from build123d import *

# Parameters (mm, degrees)
F0_W            = 40
F0_H            = 20
F1_DEPTH        = 15
F2_R            = 2.5
F3_DEPTH        = 15.001
F4_W            = 7
F4_H            = 3.5
F5_DEPTH        = 14.5
F6_W            = 4
F6_H            = 2.5
F7_DEPTH        = 12.5
F7_COPIES_COUNT = 2
F7_COPIES_PITCH = 31.5
F8_T1_DEPTH     = 2.5
F9_T4_DEPTH     = 2.5
F9_S5_R         = 2.5
F9_T6_DEPTH     = 4


# Not quite as in the source:
# - a fillet or chamfer that OpenCascade refuses, or shapes differently, is made with other operations: its cross-section is extruded or revolved along the edge and cut away or added
# - a pattern or mirror of a feature is missing from the dataset's text; its kind, count and spacing are read off the source's solid


with BuildPart() as f1:
    # F0 (on Top) → F1 (new body)
    with BuildSketch(Plane.XY):
        Rectangle(F0_W, F0_H)
    extrude(amount=F1_DEPTH)

    # F2 (on face) → F3 (cut, through all)
    with BuildSketch(Plane.XY.offset(15)):
        with Locations((-10, 0)):
            Circle(F2_R)
        with Locations((10, 0)):
            Circle(F2_R)
    extrude(amount=-F3_DEPTH, mode=Mode.SUBTRACT)

    # F4 (on face) → F5 (cut)
    with BuildSketch(Plane(origin=(-20, 0, 0), x_dir=(0, -1, 0), z_dir=(-1, 0, 0))):
        with Locations((0, 4.25)):
            Rectangle(F4_W, F4_H)
        with Locations((0, 10.75)):
            Rectangle(F4_W, F4_H)
    f5 = extrude(amount=-F5_DEPTH, mode=Mode.SUBTRACT)

    # F5_copies: F5 across plane
    add(f5.mirror(Plane(origin=(0, 0, 0), x_dir=(0, 0, 1), z_dir=(1, 0, 0))), mode=Mode.SUBTRACT)

    # F6 (on face) → F7 (cut)
    with BuildSketch(Plane(origin=(-20, 0, 0), x_dir=(0, -1, 0), z_dir=(-1, 0, 0))):
        with Locations((0, 13.75)):
            Rectangle(F6_W, F6_H)
    f7 = extrude(amount=-F7_DEPTH, mode=Mode.SUBTRACT)

    # F7_copies: F7 ×2
    with Locations(*[(i * F7_COPIES_PITCH, 0, 0) for i in range(1, F7_COPIES_COUNT)]):
        add(f7, mode=Mode.SUBTRACT)

    # F8: fillet of radius 2.5 on 1 edges, made by hand

    # F8_s2 → F8_t1 (join)
    with BuildSketch(Plane.XY.offset(12.5)):
        with BuildLine():
            ThreePointArc((-8.5, -2), (-7.7639320225, -1.1180339887), (-7.5, 0))
            Line((-7.5, 0), (-7.5, -2))
            Line((-7.5, -2), (-8.5, -2))
        make_face()
    extrude(amount=F8_T1_DEPTH)

    # F9: fillet of radius 2.5 on 1 edges, made by hand


with BuildPart() as f9_tool2:
    # F9_s3 → F9_t4 (new body)
    with BuildSketch(Plane.XY.offset(15)):
        with BuildLine():
            ThreePointArc((-7.5, -0.5), (-8.232233047, 1.267766953), (-10, 2))
            Line((-10, 2), (-7.5, 2))
            Line((-7.5, 2), (-7.5, -0.5))
        make_face()
    extrude(amount=-F9_T4_DEPTH)

    # F9_s5 → F9_t6 (cut, symmetric)
    with BuildSketch(Plane.XY.offset(13.8)):
        with Locations((-10, 0)):
            Circle(F9_S5_R)
    extrude(amount=F9_T6_DEPTH, both=True, mode=Mode.SUBTRACT)


with BuildPart() as f1_1:
    add(f1.part)

    # F9_t1: union F9_tool2
    add(f9_tool2.part)


solid = f1_1.part
CAD build for the part. Positions are in the model's coordinates, mm. A direction names the side the tool comes from. Give positions to 0.01 mm unless a question says otherwise; leave off trailing zeros. Order: outer loops, then holes, each group sorted by start corner. A loop starts at its lowest first (then second) coordinate and runs counter-clockwise, first axis right, second up. Notation, with made-up numbers: (-22.75, -30) -> (-13.75, -30) arc R21 ccw to (-13.75, -24) -> close; hole circle Ø1 at (-0.75, 75). An arc over 180 degrees is marked (long way). Return JSON: item names as keys, results as strings.
Q1. Which spindle directions (+Z, -Z, +X, -X, +Y, -Y) get a long thin tool onto all of the face, cutting with end or side? Do faces 1 (the face through (13, 3.5, 11)), 2 (the face through (-13, 3.5, 11)), 3 (the face through (7.5, 0.1, 1.3)). Say none if no direction does.
Working result:
{"face 1": "+X", "face 2": "-X", "face 3": "+Z, -Z"}
Q2. Saw through at C-C (x = 17). Write the cut outline in (y, z).
Working result:
{"outline": "(-10, 0) -> (10, 0) -> (10, 15) -> (2, 15) -> (2, 12.5) -> (3.5, 12.5) -> (3.5, 9) -> (-3.5, 9) -> (-3.5, 12.5) -> (-2, 12.5) -> (-2, 15) -> (-10, 15) -> close; hole (-3.5, 2.5) -> (3.5, 2.5) -> (3.5, 6) -> (-3.5, 6) -> close"}
Q3. Saw through at D-D (z = 14.25). Write the cut outline in (x, y), then the cut area to 3 significant figures.
Working result:
{"outline": "(-20, -10) -> (20, -10) -> (20, -2) -> (11.5, -2) arc R2.5 cw (long way) to (11.5, 2) -> (20, 2) -> (20, 10) -> (-20, 10) -> (-20, 2) -> (-11.5, 2) arc R2.5 cw (long way) to (-11.5, -2) -> (-20, -2) -> close", "area": "698 mm²"}
Q4. Saw through at B-B (z = 2). Write the cut outline in (x, y), then the cut area to 3 significant figures.
Working result:
{"outline": "(-20, -10) -> (20, -10) -> (20, 10) -> (-20, 10) -> close; hole circle Ø5 at (-10, 0); hole circle Ø5 at (10, 0)", "area": "761 mm²"}
Q5. Saw through at A-A (x = -10). Write the cut outline in (y, z).
Working result:
{"outline": "(-10, 0) -> (-2.5, 0) -> (-2.5, 2.5) -> (-3.5, 2.5) -> (-3.5, 6) -> (-2.5, 6) -> (-2.5, 9) -> (-3.5, 9) -> (-3.5, 12.5) -> (-2.5, 12.5) -> (-2.5, 15) -> (-10, 15) -> close; (2.5, 0) -> (10, 0) -> (10, 15) -> (2.5, 15) -> (2.5, 12.5) -> (3.5, 12.5) -> (3.5, 9) -> (2.5, 9) -> (2.5, 6) -> (3.5, 6) -> (3.5, 2.5) -> (2.5, 2.5) -> close"}
Q6. Flat gauge pins, fed straight in: pin 1 (1.8 mm diameter, centred on y = 0, z = 5, fed in from -X); pin 2 (3 mm diameter, centred on x = -10, y = 0, fed in from +Z); pin 3 (1 mm diameter, centred on y = -2, z = 3.5, fed in from +X). Where does each tip first touch, or does it go through?
Working result:
{"pin 1": "x = -5.5", "pin 2": "through", "pin 3": "x = 5.5"}
Q7. Drill centre lines: line 1 (Z direction, x = 11.5, y = 3); line 2 (Y direction, x = 10, z = 7.55); line 3 (Y direction, x = 15.5, z = 12). Where is each one in solid material? Low to high.
Working result:
{"line 1": "0 to 2.5, 6 to 9, 12.5 to 15", "line 2": "-10 to -2.5, 2.5 to 10", "line 3": "-10 to -3.5, 3.5 to 10"}
Q8. Mould opens along Z. For faces 4 (the face through (-13, 0, 9)), 5 (the face through (-12.5, 0.1, 7.5)), 6 (the face through (0, 0, 15)) say: pulls with the +Z half, pulls with the -Z half, needs draft (parallel to the pull), parting line crosses it, or undercut.
Working result:
{"face 4": "undercut", "face 5": "needs draft", "face 6": "pulls with the +Z half"}
